Source: CAD feature listing. Evaluate the final solid. Frame: model axes, mm. A direction names the side the tool comes from. Give positions to 0.01 mm unless a question says otherwise; leave off trailing zeros. Order: outer loops, then holes, each group sorted by start corner. A loop starts at its lowest first (then second) coordinate and runs counter-clockwise, first axis right, second up.
from build123d import *

# Parameters (mm, degrees)
F0_W     = 25.4
F0_H     = 50.8
F1_DEPTH = 2.54
F3_D     = 3.7973
F4_R     = 1.905
F5_DEPTH = 25.4
F6_R     = 1.27
F7_DEPTH = 25.4
F8_START = -25.4
F8_DEPTH = 25.4


with BuildPart() as f1:
    # F0 (on Top) → F1 (new body)
    with BuildSketch(Plane.XY):
        with Locations((12.7, 25.4)):
            Rectangle(F0_W, F0_H)
    extrude(amount=F1_DEPTH)

    # F3 (through all)
    with Locations(Plane.XY.offset(2.54)):
        with Locations((12.7, 44.45), (12.7, 6.35)):
            Hole(F3_D / 2)

    # F4 (on face) → F5 (join)
    with BuildSketch(Plane.XZ):
        with Locations((0, 1.905)):
            Circle(F4_R)
    extrude(amount=-F5_DEPTH)

    # F6 (on face) → F7 (cut, through all)
    with BuildSketch(Plane.XZ):
        with Locations((0, 1.905)):
            Circle(F6_R)
    extrude(amount=-F7_DEPTH, mode=Mode.SUBTRACT)

    # F4 (on face) → F8 (cut)
    with BuildSketch(Plane.XZ.offset(F8_START)):
        with Locations((0, 1.905)):
            Circle(F4_R)
    extrude(amount=-F8_DEPTH, mode=Mode.SUBTRACT)


solid = f1.part
(1) Section B-B, the plane y = 44.45. Return loops of the section in (x, z) (3 decimals).
(2) Section A-A, the plane y = 6.35. Return loops of the section in (x, z) (3 decimals).
(3) Section C-C, the plane x = 13.5. Return loops of the section in (y, z).
(4) Pin query (flat end, axial travel): pin 1 Ø5 at (x, y) = (21, 11) entering from +Z; pin 2 Ø1.9 at (x, z) = (0, 1) entering from +Y; pin 3 Ø1.5 at (x, z) = (0, 1.905) entering from -Y. Return the tip coordinate at first contact, or that it passes through.
(5) Section D-D, the plane z = 1.4. Return loops of the section in (x, y), plus the area to 3 significant figures.
(6) Draft query along X for faces 1 (the cylindrical face through (1.541, 37.922, 0.784)), 2 (the flat face through (13, 50.8, 1)), 3 (the cylindrical face through (14.207, 43.295, 1.252)), 4 (the cylindrical face through (13.112, 4.496, 1.252)). Return one class per face: +X half, -X half, draft (parallel to the pull), parting line (faces both ways), or undercut.
(7) Line query: line 1 along Y through (x, z) = (12.7, 0.8); line 2 along X through (y, z) = (8.5, 1.9) (3 decimals); line 3 along Z through (x, y) = (0, 13) (3 decimals). Output: solid intervals per line, ascending.
(8) Access query for faces 5 (the flat face through (13, 26, 2.54)), 6 (the flat face through (13, 26, 0)). Directions: +Z, -Z, +X, -X, +Y, -Y. A direction counts if a zero-diameter tool reaches every point of the face in a straight line with its end or side. Return the directions, or none.
Checks:
1. outline: (0, 0) - (10.801, 0) - (10.801, 2.54) - (1.796, 2.54) arc R1.905 cw to start; (14.599, 0) - (25.4, 0) - (25.4, 2.54) - (14.599, 2.54) - close
2. outline: (0, 0) - (10.801, 0) - (10.801, 2.54) - (1.796, 2.54) arc R1.905 ccw (long way) to start; (14.599, 0) - (25.4, 0) - (25.4, 2.54) - (14.599, 2.54) - close; hole circle Ø2.54 at (0, 1.905)
3. outline: (0, 0) - (4.63, 0) - (4.63, 2.54) - (0, 2.54) - close; (8.07, 0) - (42.73, 0) - (42.73, 2.54) - (8.07, 2.54) - close; (46.17, 0) - (50.8, 0) - (50.8, 2.54) - (46.17, 2.54) - close
4. pin 1: stops at z = 2.54
4. pin 2: stops at y = 25.4
4. pin 3: passes through
5. outline: (-1.84, 0) - (-1.17, 0) - (-1.17, 25.4) - (-1.84, 25.4) - close; (1.17, 0) - (25.4, 0) - (25.4, 50.8) - (1.84, 50.8) - (1.84, 25.4) - (1.17, 25.4) - close; hole circle Ø3.8 at (12.7, 6.35); hole circle Ø3.8 at (12.7, 44.45)
5. area: 1,210 mm2
6. face 1: -X half
6. face 2: draft
6. face 3: undercut
6. face 4: undercut
7. line 1: y = 0 to 4.45, 8.25 to 42.55, 46.35 to 50.8
7. line 2: x = -1.905 to -1.27, 1.27 to 25.4
7. line 3: z = 0 to 0.635, 3.175 to 3.81
8. face 5: +Z, +X, +Y, -Y
8. face 6: -Z, +X, -X, +Y, -Y
